from build123d import *

# Parameters (mm, degrees)
BASE_FLANGE1_DEPTH = 7.5
FILLET1_R          = 3


# Sheet-metal steps are written as plain solids
with BuildPart() as part:
    # Sketch1 → Base-Flange1 (new, symmetric)
    with BuildSketch(Plane.XY):
        with BuildLine():
            Line((-75, 0), (-58, 0))
            ThreePointArc((-58, 0), (-55.878679656, 0.878679656), (-55, 3))
            Line((-55, 3), (-55, 28.5))
            ThreePointArc((-55, 28.5), (-54.560660172, 29.560660172), (-53.5, 30))
            Line((-53.5, 30), (53.5, 30))
            ThreePointArc((53.5, 30), (54.560660172, 29.560660172), (55, 28.5))
            Line((55, 28.5), (55, 3))
            ThreePointArc((55, 3), (55.878679656, 0.878679656), (58, 0))
            Line((58, 0), (75, 0))
            Line((75, 0), (75, 1.5))
            Line((75, 1.5), (58, 1.5))
            ThreePointArc((58, 1.5), (56.939339828, 1.939339828), (56.5, 3))
            Line((56.5, 3), (56.5, 28.5))
            ThreePointArc((56.5, 28.5), (55.621320344, 30.621320344), (53.5, 31.5))
            Line((53.5, 31.5), (-53.5, 31.5))
            ThreePointArc((-53.5, 31.5), (-55.621320344, 30.621320344), (-56.5, 28.5))
            Line((-56.5, 28.5), (-56.5, 3))
            ThreePointArc((-56.5, 3), (-56.939339828, 1.939339828), (-58, 1.5))
            Line((-58, 1.5), (-75, 1.5))
            Line((-75, 1.5), (-75, 0))
        make_face()
    extrude(amount=BASE_FLANGE1_DEPTH, both=True)

    # Fillet1
    fillet1_edges = [part.edges().sort_by_distance(p)[0] for p in [
        (75, 0.75, -7.5),
        (-75, 0.75, -7.5),
        (75, 0.75, 7.5),
        (-75, 0.75, 7.5),
    ]]
    fillet(fillet1_edges, radius=FILLET1_R)


solid = part.part
Read the model definition and answer for the solid it produces. Units are mm, in the model's axes. A direction names the side the tool comes from. Coordinates: 2 decimals unless noted, no trailing zeros. Loops run counter-clockwise (first coordinate to the right, second up) from the corner with the lowest first, then second, coordinate; pieces in that order, holes last.
Q1. The part is cut by section C-C on x = -64.5. Write down the section's boundary in (y, z), and give its area (3 significant figures).
Q2. The mould has two halves that part along X. Classify faces 4 (the face through (-74.14, 0.74, 6.6)), 5 (the face through (-55, 16, 0)), 6 (the face through (74.14, 0.76, 6.6)): +X half, -X half, draft (parallel to the pull), parting line (faces both ways), or undercut.
Q3. Each of these flat-tipped pins is pushed along its axis until it touches: pin 1 Ø4 at (y, z) = (21, 4) entering from -X; pin 2 Ø3 at (y, z) = (5, -5.5) entering from +X; pin 3 Ø4.5 at (x, z) = (65, 1.5) entering from +Y; pin 4 Ø6 at (x, y) = (40, 26) entering from +Z. Where does it stop, or does it pass through?
Q4. The part is cut by section B-B on z = 3.25. Write down the section's boundary in (x, y), and give its area (3 significant figures).
Q5. The part is cut by section A-A on y = 19. Write down the section's boundary in (x, z).
Q6. Consider probe 1 along X at (y, z) = (17, 4.75); probe 2 along Y at (x, z) = (-17.5, -1.25); probe 3 along Y at (x, z) = (-62, 5). Determine where each line is inside the solid, lowest interval first.
Q7. Which of the six approach directions +Z, -Z, +X, -X, +Y, -Y give full straight-line access (tool end or side, diameter ignored) to faces 1 (the face through (67, 1.5, 0)), 2 (the face through (-56.5, 16, 0)), 3 (the face through (-1, 30, 0))?
Results below:
1. outline: (0, -7.5) - (1.5, -7.5) - (1.5, 7.5) - (0, 7.5) - close
1. area: 22.5 mm2
2. face 4: -X half
2. face 5: undercut
2. face 6: +X half
3. pin 1: stops at x = -56.5
3. pin 2: stops at x = 56.5
3. pin 3: stops at y = 1.5
3. pin 4: passes through
4. outline: (-75, 0) - (-58, 0) arc R3 ccw to (-55, 3) - (-55, 28.5) arc R1.5 cw to (-53.5, 30) - (53.5, 30) arc R1.5 cw to (55, 28.5) - (55, 3) arc R3 ccw to (58, 0) - (75, 0) - (75, 1.5) - (58, 1.5) arc R1.5 cw to (56.5, 3) - (56.5, 28.5) arc R3 ccw to (53.5, 31.5) - (-53.5, 31.5) arc R3 ccw to (-56.5, 28.5) - (-56.5, 3) arc R1.5 cw to (-58, 1.5) - (-75, 1.5) - close
4. area: 309 mm2
5. outline: (-56.5, -7.5) - (-55, -7.5) - (-55, 7.5) - (-56.5, 7.5) - close; (55, -7.5) - (56.5, -7.5) - (56.5, 7.5) - (55, 7.5) - close
6. probe 1: x = -56.5 to -55, 55 to 56.5
6. probe 2: y = 30 to 31.5
6. probe 3: y = 0 to 1.5
7. face 1: +Z, -Z, +X, +Y
7. face 2: +Z, -Z, -X, +Y
7. face 3: +Z, -Z, -Y
